The figure shows three views and two pictorial views of one solid part (mm, origin at its lowest corner). Answer the questions. A direction names the side the tool comes from. Coordinates: 2 decimals unless noted, no trailing zeros. Order: outer loops, then holes, each group sorted by start corner. A loop starts at its lowest first (then second) coordinate and runs counter-clockwise, first axis right, second up.
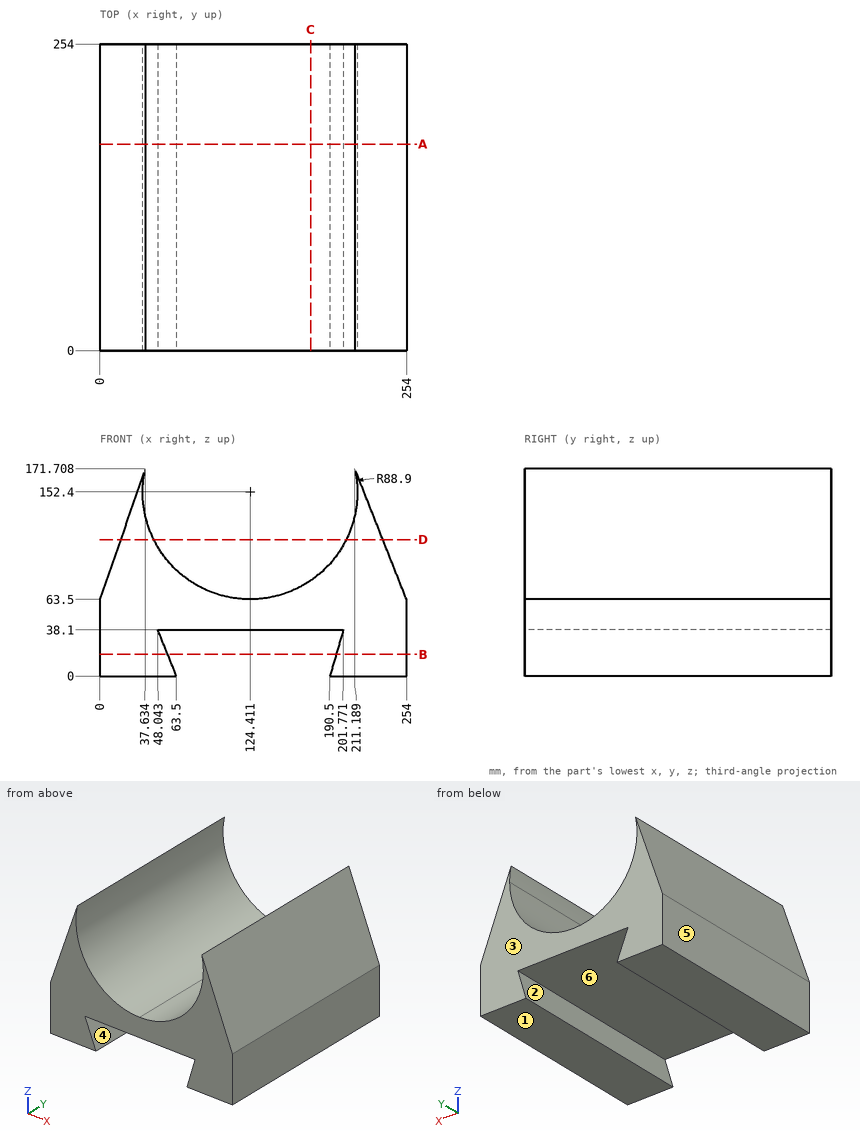
1) Straight lines are drawn through the part: probe 1 along X at (y, z) = (193.5, 79.5) (1 decimal); probe 2 along X at (y, z) = (146, 136.5) (1 decimal); probe 3 along Z at (x, y) = (76, 114.5). For each, find the intervals that lie inside material, in ascending order.
2) A cutting plane is placed at D-D, the plane z = 113. Write down the section's boundary in (x, y) (1 decimal), plus the area to 3 significant figures.
3) The mould has two halves that part along X. Classify the marked faces 3, 4, 5 and 6: released by +X, released by -X, zero draft, split by the parting line, or undercut.
4) A cutting plane is placed at C-C, the plane x = 174.5. Write down the section's boundary in (y, z), plus the area to 3 significant figures.
5) A cutting plane is placed at A-A, the plane y = 171. Write down the section's boundary in (x, z).
6) Each of these flat-tipped pins is pushed along its axis until it touches: P1, Ø6, axis at x = 173.5, y = 210.5, coming from the +Z side; P2, Ø2, axis at x = 93, z = 59, coming from the -Y side; P3, Ø3, axis at y = 194, z = 150, coming from the -X side; P4, Ø10, axis at y = 74.5, z = 149.5, coming from the +X side. Where does it stop, or does it pass through?
7) For the marked faces 1 and 2, determine the directions among +Z, -Z, +X, -X, +Y, -Y from which every point of the face is accessible in a straight line to the end or side of a thin tool.
8) A cutting plane is placed at B-B, the plane z = 18. Write down the section's boundary in (x, y) (1 decimal).
Working result:
1. probe 1: x = 5.6 to 73.5, 175.3 to 247.7
1. probe 2: x = 25.4 to 36.9, 211.9 to 225.1
1. probe 3: z = 38.1 to 77.84
2. outline: (17.2, 0) - (44.7, 0) - (44.7, 254) - (17.2, 254) - close; (204.1, 0) - (234.4, 0) - (234.4, 254) - (204.1, 254) - close
2. area: 14,700 mm2
3. face 3: zero draft
3. face 4: undercut
3. face 5: released by -X
3. face 6: undercut
4. outline: (0, 38.1) - (254, 38.1) - (254, 78.95) - (0, 78.95) - close
4. area: 10,400 mm2
5. outline: (0, 0) - (63.5, 0) - (48.04, 38.1) - (201.77, 38.1) - (190.5, 0) - (254, 0) - (254, 63.5) - (211.19, 171.71) arc R88.9 cw to (213.31, 152.4) arc R88.9 cw (long way) to (37.63, 171.71) - (0, 63.5) - close
6. P1: stops at z = 80.36
6. P2: stops at y = 0
6. P3: stops at x = 29.56
6. P4: stops at x = 221.95
7. face 1: -Z, +X, -X, +Y, -Y
7. face 2: +Y, -Y
8. outline: (0, 0) - (56.2, 0) - (56.2, 254) - (0, 254) - close; (195.8, 0) - (254, 0) - (254, 254) - (195.8, 254) - close
